Build history of the part. All positions in model axes, mm. A direction names the side the tool comes from. Give positions to 0.01 mm unless a question says otherwise; leave off trailing zeros. Order: outer loops, then holes, each group sorted by start corner. A loop starts at its lowest first (then second) coordinate and runs counter-clockwise, first axis right, second up. Notation, with made-up numbers: (-12.5, 7.5) -> (25.5, 7.5) arc R8 ccw to (25.5, 22.5) -> close; hole circle Ø1 at (3.25, -25.5). An arc over 180 degrees is marked (long way). Use a Markdown table: item, result. Add a question column.
```python
from build123d import *

# Parameters (mm, degrees)
SKETCH_1_W          = 2
SKETCH_1_H          = 2.4
EXTRUDE_1_DEPTH     = 3
SKETCH_2_W          = 11
SKETCH_2_H          = 38
CUT_EXTRUDE_1_DEPTH = 1
CUT_EXTRUDE_START   = -2
CUT_EXTRUDE_2_DEPTH = 2
SKETCH_4_R          = 1.6
CUT_EXTRUDE_3_DEPTH = 62.990079852
SKETCH_6_W          = 2.2
SKETCH_6_H          = 4
CUT_EXTRUDE_4_DEPTH = 2
SKETCH_7_R          = 4.1
CUT_EXTRUDE_5_DEPTH = 63.030395775
FILLET_1_R          = 1
CHAMFER_1_SIZE      = 0.3


with BuildPart() as part:
    # 草图1 → 凸台-拉伸1 (new body)
    with BuildSketch(Plane.XY):
        with BuildLine():
            Line((47.4, -34.9), (47.4, 34.9))
            ThreePointArc((47.4, 34.9), (45.935533906, 38.435533906), (42.4, 39.9))
            Line((42.4, 39.9), (21.6, 39.9))
            ThreePointArc((21.6, 39.9), (18.064466094, 38.435533906), (16.6, 34.9))
            Line((16.6, 34.9), (16.6, -34.9))
            ThreePointArc((16.6, -34.9), (18.064466094, -38.435533906), (21.6, -39.9))
            Line((21.6, -39.9), (42.4, -39.9))
            ThreePointArc((42.4, -39.9), (45.935533906, -38.435533906), (47.4, -34.9))
        make_face()
        with Locations((32.413843028, 28.102429875)):
            Rectangle(SKETCH_1_W, SKETCH_1_H, mode=Mode.SUBTRACT)
        with BuildLine():
            Line((40.513850359, -21.477641558), (40.513850359, -10.127641653))
            ThreePointArc((40.513850359, -10.127641653), (40.367403749, -9.774088262), (40.013850359, -9.627641653))
            Line((40.013850359, -9.627641653), (30.013850359, -9.627641653))
            ThreePointArc((30.013850359, -9.627641653), (29.660296968, -9.774088262), (29.513850359, -10.127641653))
            Line((29.513850359, -10.127641653), (29.513850359, -21.477641558))
            ThreePointArc((29.513850359, -21.477641558), (29.660296968, -21.831194949), (30.013850359, -21.977641558))
            Line((30.013850359, -21.977641558), (40.013850359, -21.977641558))
            ThreePointArc((40.013850359, -21.977641558), (40.367403749, -21.831194949), (40.513850359, -21.477641558))
        make_face(mode=Mode.SUBTRACT)
        with Locations((37.413843028, 28.102429875)):
            Rectangle(SKETCH_1_W, SKETCH_1_H, mode=Mode.SUBTRACT)
        with BuildLine():
            Line((40.464996896, 6.495389649), (40.464996896, -6.604609867))
            ThreePointArc((40.464996896, -6.604609867), (40.406418252, -6.746031223), (40.264996896, -6.804609867))
            Line((40.264996896, -6.804609867), (28.963873947, -6.804609867))
            ThreePointArc((28.963873947, -6.804609867), (28.822452591, -6.746031223), (28.763873947, -6.604609867))
            Line((28.763873947, -6.604609867), (28.763873947, 6.495389649))
            ThreePointArc((28.763873947, 6.495389649), (28.822452591, 6.636811005), (28.963873947, 6.695389649))
            Line((28.963873947, 6.695389649), (40.264996896, 6.695389649))
            ThreePointArc((40.264996896, 6.695389649), (40.406418252, 6.636811005), (40.464996896, 6.495389649))
        make_face(mode=Mode.SUBTRACT)
        with BuildLine():
            Line((40.513843009, 11.302412116), (40.513843009, 19.702429875))
            ThreePointArc((40.513843009, 19.702429875), (40.396685721, 19.985272588), (40.113843009, 20.102429875))
            Line((40.113843009, 20.102429875), (29.713821303, 20.102429875))
            ThreePointArc((29.713821303, 20.102429875), (29.43097859, 19.985272588), (29.313821303, 19.702429875))
            Line((29.313821303, 19.702429875), (29.313821303, 11.302412116))
            ThreePointArc((29.313821303, 11.302412116), (29.43097859, 11.019569403), (29.713821303, 10.902412116))
            Line((29.713821303, 10.902412116), (40.113843009, 10.902412116))
            ThreePointArc((40.113843009, 10.902412116), (40.396685721, 11.019569403), (40.513843009, 11.302412116))
        make_face(mode=Mode.SUBTRACT)
    extrude(amount=-EXTRUDE_1_DEPTH)

    # 草图2 → 切除-拉伸1 (cut)
    with BuildSketch(Plane(origin=(0, 0, -3), x_dir=(-1, 0, 0), z_dir=(0, 0, -1))):
        with Locations((-22.1, 0)):
            Rectangle(SKETCH_2_W, SKETCH_2_H)
    extrude(amount=-CUT_EXTRUDE_1_DEPTH, mode=Mode.SUBTRACT)

    # 草图3 → 切除-拉伸2 (cut)
    with BuildSketch(Plane(origin=(0, 0, -3), x_dir=(-1, 0, 0), z_dir=(0, 0, -1)).offset(CUT_EXTRUDE_START)):
        with BuildLine():
            Line((-47.4, -31.4), (-38.9, -31.4))
            Line((-38.9, -31.4), (-38.9, -39.9))
            Line((-38.9, -39.9), (-42.4, -39.9))
            ThreePointArc((-42.4, -39.9), (-45.935533906, -38.435533906), (-47.4, -34.9))
            Line((-47.4, -34.9), (-47.4, -31.4))
        make_face()
        with BuildLine():
            Line((-47.4, 34.9), (-47.4, 31.4))
            Line((-47.4, 31.4), (-38.9, 31.4))
            Line((-38.9, 31.4), (-38.9, 39.9))
            Line((-38.9, 39.9), (-42.4, 39.9))
            ThreePointArc((-42.4, 39.9), (-45.935533906, 38.435533906), (-47.4, 34.9))
        make_face()
        with BuildLine():
            Line((-16.6, 31.4), (-25.1, 31.4))
            Line((-25.1, 31.4), (-25.1, 39.9))
            Line((-25.1, 39.9), (-21.6, 39.9))
            ThreePointArc((-21.6, 39.9), (-18.064466094, 38.435533906), (-16.6, 34.9))
            Line((-16.6, 34.9), (-16.6, 31.4))
        make_face()
        with BuildLine():
            Line((-16.6, -34.9), (-16.6, -31.4))
            Line((-16.6, -31.4), (-25.1, -31.4))
            Line((-25.1, -31.4), (-25.1, -39.9))
            Line((-25.1, -39.9), (-21.6, -39.9))
            ThreePointArc((-21.6, -39.9), (-18.064466094, -38.435533906), (-16.6, -34.9))
        make_face()
    extrude(amount=CUT_EXTRUDE_2_DEPTH, mode=Mode.SUBTRACT)

    # 草图4 → 切除-拉伸3 (cut, through all)
    with BuildSketch(Plane(origin=(0, 0, -1), x_dir=(-1, 0, 0), z_dir=(0, 0, -1))):
        with Locations((-20.872307757, 35.627692243)):
            Circle(SKETCH_4_R)
        with Locations(Location((-20.872307757, -35.627692243, 0), (0, 0, 180))):
            Circle(SKETCH_4_R)
        with Locations((-43.127692243, -35.627692243)):
            Circle(SKETCH_4_R)
        with Locations(Location((-43.127692243, 35.627692243, 0), (0, 0, 180))):
            Circle(SKETCH_4_R)
    extrude(amount=-CUT_EXTRUDE_3_DEPTH, mode=Mode.SUBTRACT)

    # 草图6 → 切除-拉伸4 (cut)
    with BuildSketch(Plane(origin=(0, 0, -3), x_dir=(-1, 0, 0), z_dir=(0, 0, -1))):
        with Locations((-37.413843028, 28.102429875)):
            Rectangle(SKETCH_6_W, SKETCH_6_H)
        with Locations((-32.413843028, 28.102429875)):
            Rectangle(SKETCH_6_W, SKETCH_6_H)
    extrude(amount=-CUT_EXTRUDE_4_DEPTH, mode=Mode.SUBTRACT)

    # 草图7 → 切除-拉伸5 (cut, through all)
    with BuildSketch(Plane.XY):
        with Locations((32, -30.938820779)):
            Circle(SKETCH_7_R)
    extrude(amount=-CUT_EXTRUDE_5_DEPTH, mode=Mode.SUBTRACT)

    # 圆角1
    fillet_1_edges = [part.edges().sort_by_distance(p)[0] for p in [
        (25.1, -39.9, -2),
        (16.6, -31.4, -2),
        (16.6, 31.4, -2),
        (25.1, 39.9, -2),
        (38.9, 39.9, -2),
        (47.4, 31.4, -2),
        (47.4, -31.4, -2),
        (38.9, -39.9, -2),
    ]]
    fillet(fillet_1_edges, radius=FILLET_1_R)

    # 倒角1
    chamfer_1_edges = [part.edges().sort_by_distance(p)[0] for p in [
        (36.413843028, 28.102429875, 0),
        (37.413843028, 26.902429875, 0),
        (38.413843028, 28.102429875, 0),
        (37.413843028, 29.302429875, 0),
        (32.413843028, 29.302429875, 0),
        (31.413843028, 28.102429875, 0),
        (32.413843028, 26.902429875, 0),
        (33.413843028, 28.102429875, 0),
    ]]
    chamfer(chamfer_1_edges, length=CHAMFER_1_SIZE)


solid = part.part
```
(1) Pin check, flat tips, straight feed: pin 1 Ø7.5 at (x, y) = (21.5, -33.5) entering from -Z; pin 2 Ø0.6 at (x, z) = (41, -2) entering from +Y; pin 3 Ø1 at (x, z) = (25, -2) entering from +Y; pin 4 Ø0.6 at (y, z) = (-36, -2) entering from -X. Stop position of each tip, or through.
(2) Band-saw the part on A-A on y = 13. Give the cut face in (x, z), plus the area to 3 significant figures.
(3) Wall check: probe 1 along Y at (x, z) = (32, -0.85); probe 2 along Y at (x, z) = (38.5, -0.35); probe 3 along Y at (x, z) = (36.5, -1.8). Give the ranges that are in metal, low to high.
(4) Mould opens along Y. For faces 1 (the face through (18.03, -38.4, -0.49)), 2 (the face through (20, 34, -1)), 3 (the face through (37, 30.102, -2)) say: released by +Y, released by -Y, zero draft, split by the parting line, or undercut.
(5) Tool access for faces 4 (the face through (20, -34, -1)), 5 (the face through (22, 0, -2)), 6 (the face through (32, 30.102, -2)), 7 (the face through (35, 10.902, -1)): list every direction of +Z, -Z, +X, -X, +Y, -Y with a clear straight run to the whole face (end or side of a thin tool).
(6) Band-saw the part on B-B on y = -29. Give the cut face in (x, z), plus the area to 3 significant figures.
Response:
| question | item | result |
|---|---|---|
| 1 | pin 1 | stops at z = -3 |
| 1 | pin 2 | stops at y = 31.4 |
| 1 | pin 3 | stops at y = 39.7 |
| 1 | pin 4 | stops at x = 25.1 |
| 2 | outline | (16.6, -2) -> (27.6, -2) -> (27.6, -3) -> (29.31, -3) -> (29.31, 0) -> (16.6, 0) -> close; (40.51, -3) -> (47.4, -3) -> (47.4, 0) -> (40.51, 0) -> close |
| 2 | area | 47.8 mm² |
| 3 | probe 1 | y = -39.9 to -35.04, -26.84 to -21.98, -9.63 to -6.8, 6.7 to 10.9, 20.1 to 26.9, 29.3 to 39.9 |
| 3 | probe 2 | y = -39.9 to -21.98, -9.63 to -6.8, 6.7 to 10.9, 20.1 to 39.9 |
| 3 | probe 3 | y = -39.9 to -21.98, -9.63 to -6.8, 6.7 to 10.9, 20.1 to 26.1, 30.1 to 39.9 |
| 4 | face 1 | released by -Y |
| 4 | face 2 | zero draft |
| 4 | face 3 | undercut |
| 5 | face 4 | -Z, -X, -Y |
| 5 | face 5 | -Z, -X |
| 5 | face 6 | -Z |
| 5 | face 7 | +Z, -Z |
| 6 | outline | (16.6, -3) -> (28.39, -3) -> (28.39, 0) -> (16.6, 0) -> close; (35.61, -3) -> (47.4, -3) -> (47.4, 0) -> (35.61, 0) -> close |
| 6 | area | 70.7 mm² |
